Input: dimensioned drawing with shaded views. Units: mm. Origin: part minimum x, y, z. A direction names the side the tool comes from. Round coordinates to 2 decimals unless told otherwise and drop trailing zeros. Loops run counter-clockwise (first coordinate to the right, second up) from the corner with the lowest first, then second, coordinate; pieces in that order, holes last.
1) Access query for the marked faces 5 and 6. Directions: +Z, -Z, +X, -X, +Y, -Y. A direction counts if a zero-diameter tool reaches every point of the face in a straight line with its end or side. Return the directions, or none.
2) Section D-D, the plane z = 13.75. Return loops of the section in (x, y), and give its area (3 significant figures).
3) Section A-A, the plane y = 12. Return loops of the section in (x, z).
4) Section C-C, the plane x = 19.5. Return loops of the section in (y, z).
5) Draft query along Y for the marked faces 1, 2, 3 and 4. Return one class per face: pulls with the +Y half, pulls with the -Y half, needs draft (parallel to the pull), parting line crosses it, or undercut.
6) Section B-B, the plane z = 6.5. Return loops of the section in (x, y), and give its area (3 significant figures).
7) Ray query, line 1 along X through (y, z) = (16, 3.5); line 2 along Y through (x, z) = (4.25, 1.75). Return the intervals inside material, ascending.
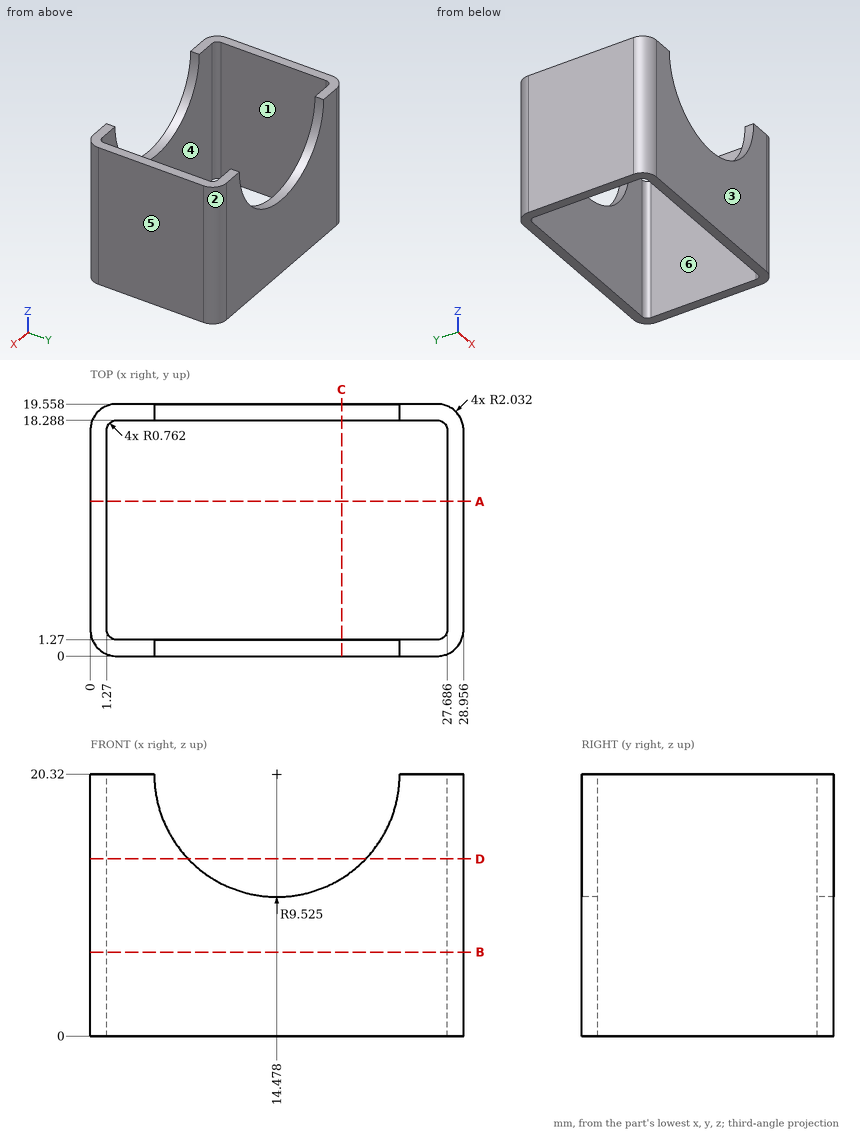
Final values:
1. face 5: +Z, -Z, +X, +Y, -Y
1. face 6: +Z, -Z
2. outline: (0, 2.03) arc R2.03 ccw to (2.03, 0) - (7.58, 0) - (7.58, 1.27) - (2.03, 1.27) arc R0.76 cw to (1.27, 2.03) - (1.27, 17.53) arc R0.76 cw to (2.03, 18.29) - (7.58, 18.29) - (7.58, 19.56) - (2.03, 19.56) arc R2.03 ccw to (0, 17.53) - close; (21.37, 0) - (26.92, 0) arc R2.03 ccw to (28.96, 2.03) - (28.96, 17.53) arc R2.03 ccw to (26.92, 19.56) - (21.37, 19.56) - (21.37, 18.29) - (26.92, 18.29) arc R0.76 cw to (27.69, 17.53) - (27.69, 2.03) arc R0.76 cw to (26.92, 1.27) - (21.37, 1.27) - close
2. area: 78.7 mm2
3. outline: (0, 0) - (1.27, 0) - (1.27, 20.32) - (0, 20.32) - close; (27.69, 0) - (28.96, 0) - (28.96, 20.32) - (27.69, 20.32) - close
4. outline: (0, 0) - (1.27, 0) - (1.27, 12.23) - (0, 12.23) - close; (18.29, 0) - (19.56, 0) - (19.56, 12.23) - (18.29, 12.23) - close
5. face 1: undercut
5. face 2: pulls with the +Y half
5. face 3: pulls with the -Y half
5. face 4: undercut
6. outline: (0, 2.03) arc R2.03 ccw to (2.03, 0) - (26.92, 0) arc R2.03 ccw to (28.96, 2.03) - (28.96, 17.53) arc R2.03 ccw to (26.92, 19.56) - (2.03, 19.56) arc R2.03 ccw to (0, 17.53) - close; hole (1.27, 2.03) arc R0.76 ccw to (2.03, 1.27) - (26.92, 1.27) arc R0.76 ccw to (27.69, 2.03) - (27.69, 17.53) arc R0.76 ccw to (26.92, 18.29) - (2.03, 18.29) arc R0.76 ccw to (1.27, 17.53) - close
6. area: 114 mm2
7. line 1: x = 0 to 1.27, 27.69 to 28.96
7. line 2: y = 0 to 1.27, 18.29 to 19.56
